Solid Edge part; units mm, degrees
sketch "Sketch1" plane through (0, 0, 0) normal (0, -1, 0) x (1, 0, 0)
  line L0 (-5, 25) -> (-5, 19)
  line L1 (5, 19) -> (-5, 19)
  line L2 (5, 35) -> (5, 19)
  line L3 (5, 35) -> (-90, 35)
  line L4 (-90, 35) -> (-100, 25)
  line L5 (-100, 25) -> (-100, 10)
  line L6 (-100, 10) -> (-90, 10)
  line L7 (-90, 10) -> (-90, 20.8579)
  line L8 (-90, 20.8579) -> (-85.8579, 25)
  line L9 (-85.8579, 25) -> (-45, 25)
  line L10 (-45, 25) -> (-45, 5)
  arc A0 (-35, 5) -> (-45, 5) centre (-40, 5) cw
  line L11 (-35, 5) -> (-35, 25)
  line L12 (-35, 25) -> (-5, 25)
  dimension "D1" = 35
extrude "Protrusion1" add sketch "Sketch1" along normal mid plane 10
fillet "Round_1" radius 5 4 edges at (-5, -5, 22) (-5, 5, 22) (5, 5, 27) (5, -5, 27)
sketch "Sketch2" plane through (0, 0, 0) normal (0, -1, 0) x (1, 0, 0)
  circle A0 centre (-80, 30) radius 1.35
extrude "ExtrudedCutout_3" cut sketch "Sketch2" along normal mid plane 29.2691
sketch "Sketch3" plane through (-100, 0, 15) normal (-1, 0, 0) x (0, 0, -1)
  line L0 (5, 2.5) -> (0, 2.5)
  line L1 (0, 2.5) -> (0, -2.5)
  line L2 (0, -2.5) -> (5, -2.5)
  line L3 (5, -2.5) -> (5, 2.5)
  dimension "D1" = 5
extrude "ExtrudedCutout_4" cut sketch "Sketch3" against normal blind 5
fillet "Round_6" radius 2 1 edges at (-100, 2.5, 12.5)
hole "Hole_1" at (-40, -5, 5) direction (0, 1, 0) diameter 4.5 end up to next
fillet "Round_7" radius 5 2 edges at (-45, 0, 25) (-35, 0, 25)
chamfer "Chamfer_4" distance 3.4 angle 60 1 edges at (-5, 0, 19) measured on face at (3.4333, -3.2333, 19)
properties material "PVC"
Here's how the part is built. I have some questions about the finished solid (model axes, mm). A direction names the side the tool comes from. Coordinates: 2 decimals unless noted, no trailing zeros. Loops run counter-clockwise (first coordinate to the right, second up) from the corner with the lowest first, then second, coordinate; pieces in that order, holes last. Notation, with made-up numbers: M -20,-27 L 8,-27 A14 cw 8,-3 Z; hole C -28,54 d2. An arc over 180 degrees is marked long. One line per item, written item: value.
1. Imagine slicing it at A-A (x = -80). List the corners of the cut face in (y, z) for me, and give its area (3 significant figures).
Geometry says:
outline: M -5,25 L 5,25 L 5,28.65 L -5,28.65 Z; M -5,31.35 L 5,31.35 L 5,35 L -5,35 Z
area: 73.0 mm2
2. Please list where these lines run through material, in increasing order: probe 1 along X at (y, z) = (2.25, 13); probe 2 along X at (y, z) = (2.5, 5); probe 3 along X at (y, z) = (-0.75, 20.5).
Geometry says:
probe 1: x = -95 to -90, -45 to -35
probe 2: x = -45 to -42.25, -37.75 to -35
probe 3: x = -100 to -90, -45.03 to -34.97, -2.35 to 2.35
3. Imagine slicing it at C-C (z = 22). State how many separate pieces and enclosed holes the cut face has, and give its area (3 significant figures).
Geometry says:
separate pieces: 3
enclosed holes: 0
area: 255 mm2
4. Thinking about a two-plate mould opening in X: for faces 1 (the conical face through (-2.376, -2.324, 21.986)), 2 (the flat face through (-95, 0, 13)), 3 (the flat face through (-42, 0, 35)), which applies, +X half, -X half, draft (parallel to the pull), parting line (faces both ways), or undercut?
Geometry says:
face 1: undercut
face 2: -X half
face 3: draft
5. Will these pins go through, and if not, where does the flat tip stop? pin 1 Ø4.5 at (x, z) = (-80, 30) entering from +Y; pin 2 Ø5 at (y, z) = (-2.5, 6) entering from +X; pin 3 Ø5 at (x, y) = (-21, 0.5) entering from -Z; pin 4 Ø5.5 at (x, y) = (-98, 0.5) entering from -Z.
Geometry says:
pin 1: stops at y = 5
pin 2: stops at x = -35
pin 3: stops at z = 25
pin 4: stops at z = 10
6. On a 3-axis mill with a long thin cutter (end or side, diameter ignored), from which of +Z, -Z, +X, -X, +Y, -Y can I reach the whole of each face in a straight line? I mean faces 4 (the flat face through (-68, 0, 25)), 5 (the cylindrical face through (3, 4, 30)), 6 (the flat face through (-94, 0, 10)), 7 (the flat face through (-97, 2.5, 13)). Say none if no direction works.
Geometry says:
face 4: -Z, +Y, -Y
face 5: +Z, -Z, +X, +Y
face 6: -Z, -X, +Y, -Y
face 7: -Z, -X
7. Imagine slicing it at D-D (x = -40). List the corners of the cut face in (y, z) for me, and give its area (3 significant figures).
Geometry says:
outline: M -5,0 L 5,0 L 5,2.75 L -5,2.75 Z; M -5,7.25 L 5,7.25 L 5,35 L -5,35 Z
area: 305 mm2
